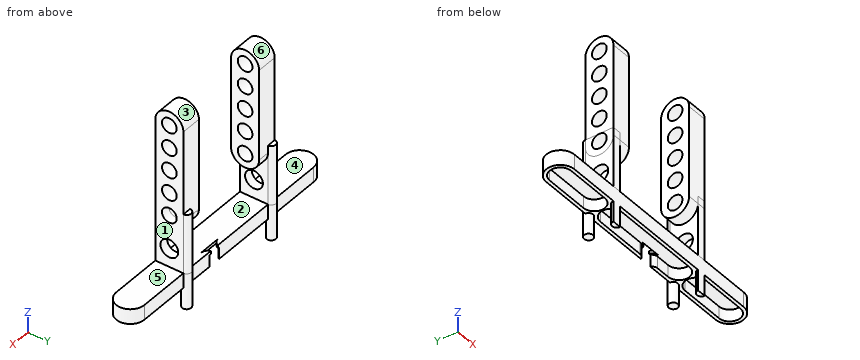
```python
from build123d import *

# Parameters (mm, degrees)
EXTRUDE_1_DEPTH          = 2
EXTRUDE_START            = -24
SKETCH_2_R               = 3
EXTRUDE_2_DEPTH          = 24
EXTRUDE_START_2          = 8
EXTRUDE_3_DEPTH          = 8
SKETCH_5_W               = 143.526768474
SKETCH_5_H               = 22.779611496
CUT_EXTRUDE_1_DEPTH      = 90.927438057
EXTRUDE_4_DEPTH          = 50
SKETCH_7_R               = 6
CUT_EXTRUDE_2_DEPTH      = 138.469699072
SKETCH_8_W               = 162.700191743
SKETCH_8_H               = 85.823894635
CUT_EXTRUDE_3_DEPTH      = 10
SKETCH_9_R               = 4.95
EXTRUDE_5_DEPTH          = 14
EXTRUDE_START_3          = -14
SKETCH_10_R              = 4.95
EXTRUDE_6_DEPTH          = 14
CUT_EXTRUDE_4_DEPTH      = 157.127849217
CUT_EXTRUDE_4_DEPTH_BACK = 157.127849217
SKETCH_11_R              = 4.95


with BuildPart() as part:
    # Эскиз1 → Бобышка-Вытянуть1 (new body)
    with BuildSketch(Plane.XY):
        with BuildLine():
            Line((20.999794095, 5.325), (5.329794095, 5.325))
            ThreePointArc((5.329794095, 5.325), (8.180232657, 6.217080819), (10.013542594, 8.575))
            Line((10.013542594, 8.575), (-35.092602953, 8.575))
            ThreePointArc((-35.092602953, 8.575), (-38.092602953, 5.575), (-41.092602953, 8.575))
            Line((-41.092602953, 8.575), (-76.185205905, 8.575))
            ThreePointArc((-76.185205905, 8.575), (-85.635205905, -0.875), (-76.185205905, -10.325))
            Line((-76.185205905, -10.325), (-41.092602953, -10.325))
            ThreePointArc((-41.092602953, -10.325), (-38.092602953, -7.325), (-35.092602953, -10.325))
            Line((-35.092602953, -10.325), (35.092602953, -10.325))
            ThreePointArc((35.092602953, -10.325), (38.092602953, -7.325), (41.092602953, -10.325))
            Line((41.092602953, -10.325), (76.185205905, -10.325))
            ThreePointArc((76.185205905, -10.325), (85.635205905, -0.875), (76.185205905, 8.575))
            Line((76.185205905, 8.575), (41.092602953, 8.575))
            ThreePointArc((41.092602953, 8.575), (38.092602953, 5.575), (35.092602953, 8.575))
            Line((35.092602953, 8.575), (16.316045596, 8.575))
            ThreePointArc((16.316045596, 8.575), (18.149355532, 6.217080819), (20.999794095, 5.325))
        make_face()
    extrude(amount=EXTRUDE_1_DEPTH)

    # Эскиз2 → Бобышка-Вытянуть2 (add)
    with BuildSketch(Plane.XY.offset(2).offset(EXTRUDE_START)):
        with Locations(Location((38.092602953, 8.575, 0), (0, 0, 180))):
            Circle(SKETCH_2_R)
        with Locations(Location((38.092602953, -10.325, 0), (0, 0, 180))):
            Circle(SKETCH_2_R)
        with Locations(Location((-38.092602953, -10.325, 0), (0, 0, 180))):
            Circle(SKETCH_2_R)
        with Locations(Location((-38.092602953, 8.575, 0), (0, 0, 180))):
            Circle(SKETCH_2_R)
    extrude(amount=EXTRUDE_2_DEPTH)

    # Эскиз4 → Бобышка-Вытянуть3 (add)
    with BuildSketch(Plane(origin=(0, 0, 0), x_dir=(-1, 0, 0), z_dir=(0, 0, -1)).offset(EXTRUDE_START_2)):
        with BuildLine():
            Line((-17.402920452, 8.575), (-35.092602953, 8.575))
            ThreePointArc((-35.092602953, 8.575), (-38.092602953, 5.575), (-41.092602953, 8.575))
            Line((-41.092602953, 8.575), (-76.185205905, 8.575))
            ThreePointArc((-76.185205905, 8.575), (-85.635205905, -0.875), (-76.185205905, -10.325))
            Line((-76.185205905, -10.325), (-41.092602953, -10.325))
            ThreePointArc((-41.092602953, -10.325), (-38.092602953, -7.325), (-35.092602953, -10.325))
            Line((-35.092602953, -10.325), (35.092602953, -10.325))
            ThreePointArc((35.092602953, -10.325), (38.092602953, -7.325), (41.092602953, -10.325))
            Line((41.092602953, -10.325), (76.185205905, -10.325))
            ThreePointArc((76.185205905, -10.325), (85.635205905, -0.875), (76.185205905, 8.575))
            Line((76.185205905, 8.575), (41.092602953, 8.575))
            ThreePointArc((41.092602953, 8.575), (38.092602953, 5.575), (35.092602953, 8.575))
            Line((35.092602953, 8.575), (-8.926667737, 8.575))
            ThreePointArc((-8.926667737, 8.575), (-7.451114438, 6.933835008), (-5.329794095, 6.325))
            Line((-5.329794095, 6.325), (30.474082362, 6.325))
            ThreePointArc((30.474082362, 6.325), (37.674082362, -0.875), (30.474082362, -8.075))
            Line((30.474082362, -8.075), (-30.474082362, -8.075))
            ThreePointArc((-30.474082362, -8.075), (-37.674082362, -0.875), (-30.474082362, 6.325))
            Line((-30.474082362, 6.325), (-20.999794095, 6.325))
            ThreePointArc((-20.999794095, 6.325), (-18.878473751, 6.933835008), (-17.402920452, 8.575))
        make_face()
        with BuildLine():
            Line((-45.711123543, 6.325), (-76.185205905, 6.325))
            ThreePointArc((-76.185205905, 6.325), (-83.385205905, -0.875), (-76.185205905, -8.075))
            Line((-76.185205905, -8.075), (-45.711123543, -8.075))
            ThreePointArc((-45.711123543, -8.075), (-38.511123543, -0.875), (-45.711123543, 6.325))
        make_face(mode=Mode.SUBTRACT)
        with BuildLine():
            Line((76.185205905, 6.325), (45.711123543, 6.325))
            ThreePointArc((45.711123543, 6.325), (38.511123543, -0.875), (45.711123543, -8.075))
            Line((45.711123543, -8.075), (76.185205905, -8.075))
            ThreePointArc((76.185205905, -8.075), (83.385205905, -0.875), (76.185205905, 6.325))
        make_face(mode=Mode.SUBTRACT)
    extrude(amount=-EXTRUDE_3_DEPTH)

    # Эскиз5 → Вырез-Вытянуть1 (cut, through all)
    with BuildSketch(Plane.XY.offset(2)):
        with Locations((16.343060787, -21.714805748)):
            Rectangle(SKETCH_5_W, SKETCH_5_H)
    extrude(amount=-CUT_EXTRUDE_1_DEPTH, mode=Mode.SUBTRACT)

    # Эскиз6 → Бобышка-Вытянуть4 (add)
    with BuildSketch(Plane.XY.offset(2)):
        with BuildLine():
            ThreePointArc((-35.092602953, 8.575), (-38.092602953, 11.575), (-41.092602953, 8.575))
            Line((-41.092602953, 8.575), (-41.092602953, -10.325))
            Line((-41.092602953, -10.325), (-35.092602953, -10.325))
            Line((-35.092602953, -10.325), (-35.092602953, 8.575))
        make_face()
        with BuildLine():
            Line((35.092602953, 8.575), (35.092602953, -10.325))
            Line((35.092602953, -10.325), (41.092602953, -10.325))
            Line((41.092602953, -10.325), (41.092602953, 8.575))
            ThreePointArc((41.092602953, 8.575), (38.092602953, 11.575), (35.092602953, 8.575))
        make_face()
    extrude(amount=EXTRUDE_4_DEPTH)

    # Эскиз7 → Вырез-Вытянуть2 (cut, through all)
    with BuildSketch(Plane(origin=(41.092602953, 0, 0), x_dir=(0, 0, -1), z_dir=(1, 0, 0))):
        with Locations(Location((-14.5, -0.875, 0), (0, 0, 90))):
            Circle(SKETCH_7_R)
    extrude(amount=-CUT_EXTRUDE_2_DEPTH, mode=Mode.SUBTRACT)

    # Эскиз8 → Вырез-Вытянуть3 (cut)
    with BuildSketch(Plane.XY.offset(52)):
        with Locations((-1.826040312, 7.472651168)):
            Rectangle(SKETCH_8_W, SKETCH_8_H)
    extrude(amount=-CUT_EXTRUDE_3_DEPTH, mode=Mode.SUBTRACT)

    # Эскиз9 → Бобышка-Вытянуть5 (add)
    with BuildSketch(Plane(origin=(41.092602953, 0, 0), x_dir=(0, 0, -1), z_dir=(1, 0, 0))):
        with BuildLine():
            Line((-97.948164724, 8.575), (-37, 8.575))
            ThreePointArc((-37, 8.575), (-27.55, -0.875), (-37, -10.325))
            Line((-37, -10.325), (-97.948164724, -10.325))
            ThreePointArc((-97.948164724, -10.325), (-107.398164724, -0.875), (-97.948164724, 8.575))
        make_face()
        with Locations(Location((-97.948164724, -0.875, 0), (0, 0, 90))):
            Circle(SKETCH_9_R, mode=Mode.SUBTRACT)
        with Locations(Location((-82.711123543, -0.875, 0), (0, 0, 90))):
            Circle(SKETCH_9_R, mode=Mode.SUBTRACT)
        with Locations(Location((-67.474082362, -0.875, 0), (0, 0, 90))):
            Circle(SKETCH_9_R, mode=Mode.SUBTRACT)
        with Locations(Location((-52.237041181, -0.875, 0), (0, 0, 90))):
            Circle(SKETCH_9_R, mode=Mode.SUBTRACT)
        with Locations(Location((-37, -0.875, 0), (0, 0, 90))):
            Circle(SKETCH_9_R, mode=Mode.SUBTRACT)
    extrude(amount=-EXTRUDE_5_DEPTH)

    # Эскиз10 → Бобышка-Вытянуть6 (add)
    with BuildSketch(Plane.ZY.offset(41.092602953).offset(EXTRUDE_START_3)):
        with BuildLine():
            Line((97.948164724, 8.575), (37, 8.575))
            ThreePointArc((37, 8.575), (27.55, -0.875), (37, -10.325))
            Line((37, -10.325), (97.948164724, -10.325))
            ThreePointArc((97.948164724, -10.325), (107.398164724, -0.875), (97.948164724, 8.575))
        make_face()
        with Locations(Location((52.237041181, -0.875, 0), (0, 0, 90))):
            Circle(SKETCH_10_R, mode=Mode.SUBTRACT)
        with Locations(Location((67.474082362, -0.875, 0), (0, 0, 90))):
            Circle(SKETCH_10_R, mode=Mode.SUBTRACT)
        with Locations(Location((82.711123543, -0.875, 0), (0, 0, 90))):
            Circle(SKETCH_10_R, mode=Mode.SUBTRACT)
        with Locations(Location((97.948164724, -0.875, 0), (0, 0, 90))):
            Circle(SKETCH_10_R, mode=Mode.SUBTRACT)
    extrude(amount=EXTRUDE_6_DEPTH)

    # Эскиз11 → Вырез-Вытянуть4 (cut, two sides: drawn at the far end of the back side and taken through both)
    with BuildSketch(Plane.ZY.offset(-27.092602953).offset(-CUT_EXTRUDE_4_DEPTH_BACK)):
        with Locations(Location((37, -0.875, 0), (0, 0, 90))):
            Circle(SKETCH_11_R)
    extrude(amount=CUT_EXTRUDE_4_DEPTH + CUT_EXTRUDE_4_DEPTH_BACK, mode=Mode.SUBTRACT)


solid = part.part
```
Input: part model. Units: mm. Frame: model coordinates. Face numbers are marked on the shaded views. A direction names the side the tool comes from. Give positions to 0.01 mm unless a question says otherwise; leave off trailing zeros. Order: outer loops, then holes, each group sorted by start corner. A loop starts at its lowest first (then second) coordinate and runs counter-clockwise, first axis right, second up. Notation, with made-up numbers: M 51,50.5 L 64,50.5 A18 cw 64,70.5 Z; hole C 35.25,4 d10. An arc over 180 degrees is marked long. Return JSON: item names as keys, results as strings.
Item 1: Pull-direction query (Z, two-part tool) for the marked faces 1, 2 and 3; classes: +Z half, -Z half, draft (parallel to the pull), parting line (faces both ways), or undercut.
Solutions:
{"face 1": "draft", "face 2": "undercut", "face 3": "+Z half"}
Item 2: Ray query, probe 1 along X at (y, z) = (-6.5, 43.5); probe 2 along X at (y, z) = (5.5, 9); probe 3 along Y at (x, z) = (-23, -5) (3 decimals). Return the intervals inside material, ascending.
Solutions:
{"probe 1": "-41.09 to -27.09, 27.09 to 41.09", "probe 2": "-41.09 to -35.09, 35.09 to 41.09", "probe 3": "-10.325 to -8.075, 6.325 to 8.575"}
Item 3: Access query for the marked faces 4, 5 and 6. Directions: +Z, -Z, +X, -X, +Y, -Y. A direction counts if a zero-diameter tool reaches every point of the face in a straight line with its end or side. Return the directions, or none.
Solutions:
{"face 4": "+Z, -X, +Y, -Y", "face 5": "+Z, +X, +Y, -Y", "face 6": "+Z, +X, -X"}
Item 4: Cut plane D-D (y = 0.75). State how many separate pieces and enclosed holes the cut face has, then the cut area to 3 significant figures.
Solutions:
{"separate pieces": "13", "enclosed holes": "0", "area": "1,490 mm^2"}
Item 5: Cut plane C-C (x = -50). Return loops of the section in (y, z) (3 decimals).
Solutions:
{"outline": "M -10.325,-8 L -8.075,-8 L -8.075,0 L 6.325,0 L 6.325,-8 L 8.575,-8 L 8.575,2 L -10.325,2 Z"}
Item 6: First-contact query: P1, Ø6, axis at y = -4, z = 11, coming from the -X side; P2, Ø5, axis at x = 23, z = -4.5, coming from the +Y side (3 decimals); P3, Ø1, axis at x = -20, y = -5.5, coming from the +Z side. Flat tips, straight axial feed; report the tip coordinate or a pass-through.
Solutions:
{"P1": "x = -41.09", "P2": "y = 8.575", "P3": "z = 2"}
Item 7: Cut plane B-B (z = 14.5). Return loops of the section in (x, y) (3 decimals), then the cut area to 3 significant figures.
Solutions:
{"outline": "M -41.093,-10.325 L -35.093,-10.325 L -35.093,-6.875 L -41.093,-6.875 Z; M -41.093,5.125 L -35.093,5.125 L -35.093,8.575 A3 ccw -41.093,8.575 Z; M 35.093,-10.325 L 41.093,-10.325 L 41.093,-6.875 L 35.093,-6.875 Z; M 35.093,5.125 L 41.093,5.125 L 41.093,8.575 A3 ccw 35.093,8.575 Z", "area": "111 mm^2"}
Item 8: Cut plane A-A (z = 76). Return loops of the section in (x, y) (3 decimals).
Solutions:
{"outline": "M -41.093,-10.325 L -27.093,-10.325 L -27.093,8.575 L -41.093,8.575 Z; M 27.093,-10.325 L 41.093,-10.325 L 41.093,8.575 L 27.093,8.575 Z"}
